Verification items for the finished model (mm, model axes). A direction names the side the tool comes from. Round coordinates to 2 decimals unless told otherwise and drop trailing zeros. Order: outer loops, then holes, each group sorted by start corner. A loop starts at its lowest first (then second) coordinate and runs counter-clockwise, first axis right, second up. Notation, with made-up numbers: (73.25, 11.25) -> (114.25, 11.25) arc R7 ccw to (114.25, 23.25) -> close; hole circle Ø4 at (-23, 53). An arc over 180 degrees is marked (long way). Put each result on its own line as item: value.
```python
from build123d import *

# Parameters (mm, degrees)
SKETCH1_R           = 2.286
BOSS_EXTRUDE1_DEPTH = 6.35
CHAMFER1_SIZE       = 15.24
CHAMFER1_SIZE2      = 24.085722971
FILLET1_R           = 3.81


with BuildPart() as part:
    # Sketch1 → Boss-Extrude1 (new body)
    with BuildSketch(Plane.XY):
        Polygon((-6.35, 31.75), (-6.35, 10.18883388), (-34.206786825, -8.403439207), (-27.156560793, -18.966786825), (-6.35, -5.08), (6.35, -5.08), (6.35, 31.75), align=None)
        Circle(SKETCH1_R, mode=Mode.SUBTRACT)
        with Locations((0, 25.4)):
            Circle(SKETCH1_R, mode=Mode.SUBTRACT)
        with Locations((-25.4, -10.16)):
            Circle(SKETCH1_R, mode=Mode.SUBTRACT)
        with Locations((0, 12.7)):
            Circle(SKETCH1_R, mode=Mode.SUBTRACT)
    extrude(amount=BOSS_EXTRUDE1_DEPTH)

    # Chamfer1
    chamfer1_edges = [part.edges().sort_by_distance(p)[0] for p in [
        (-6.35, 10.18883388, 3.175),
    ]]
    chamfer1_side = [part.faces().sort_by_distance(p)[0] for p in [
        (-6.35, 20.96941694, 3.175),
    ]]
    chamfer(chamfer1_edges, length=CHAMFER1_SIZE, length2=CHAMFER1_SIZE2, reference=chamfer1_side[0])

    # Fillet1
    fillet1_edges = [part.edges().sort_by_distance(p)[0] for p in [
        (6.35, 31.75, 3.175),
        (6.35, -5.08, 3.175),
        (-6.35, -5.08, 3.175),
        (-27.156560793, -18.966786825, 3.175),
        (-34.206786825, -8.403439207, 3.175),
        (-6.35, 31.75, 3.175),
        (-26.383532628, -3.182015811, 3.175),
        (-6.35, 25.42883388, 3.175),
    ]]
    fillet(fillet1_edges, radius=FILLET1_R)


solid = part.part
```
Item 1: Sectioned sample at C-C, the plane y = -10.16. Record the boundary of the cut face in (x, z), then the cut area to 3 significant figures.
Geometry check:
outline: (-32.67, 0) -> (-27.69, 0) -> (-27.69, 6.35) -> (-32.67, 6.35) -> close; (-23.11, 0) -> (-13.96, 0) -> (-13.96, 6.35) -> (-23.11, 6.35) -> close
area: 89.8 mm2
Item 2: Sectioned sample at A-A, the plane x = 0. Record the boundary of the cut face in (y, z), then the cut area to 3 significant figures.
Geometry check:
outline: (-5.08, 0) -> (-2.29, 0) -> (-2.29, 6.35) -> (-5.08, 6.35) -> close; (2.29, 0) -> (10.41, 0) -> (10.41, 6.35) -> (2.29, 6.35) -> close; (14.99, 0) -> (23.11, 0) -> (23.11, 6.35) -> (14.99, 6.35) -> close; (27.69, 0) -> (31.75, 0) -> (31.75, 6.35) -> (27.69, 6.35) -> close
area: 147 mm2
Item 3: Sectioned sample at B-B, the plane z = 2.25. Record the boundary of the cut face in (x, y), then the cut area to 3 significant figures.
Geometry check:
outline: (-32.09, -11.57) -> (-29.27, -15.8) arc R3.81 ccw to (-23.99, -16.85) -> (-7.31, -5.72) arc R3.81 cw to (-5.2, -5.08) -> (2.54, -5.08) arc R3.81 ccw to (6.35, -1.27) -> (6.35, 27.94) arc R3.81 ccw to (2.54, 31.75) -> (-2.54, 31.75) arc R3.81 ccw to (-6.35, 27.94) -> (-6.35, 26.63) arc R3.81 cw to (-7.04, 24.44) -> (-25.97, -2.6) arc R3.81 cw to (-26.98, -3.58) -> (-31.04, -6.29) arc R3.81 ccw to start; hole circle Ø4.57 at (-25.4, -10.16); hole circle Ø4.57 at (0, 0); hole circle Ø4.57 at (0, 12.7); hole circle Ø4.57 at (0, 25.4)
area: 911 mm2
Item 4: Material ranges on line 1 along Y through (x, z) = (0, 4.75); line 2 along Y through (x, z) = (1, 4); line 3 along X through (y, z) = (27, 0.5), recorded low to high.
Geometry check:
line 1: -5.08 to -2.29, 2.29 to 10.41, 14.99 to 23.11, 27.69 to 31.75
line 2: -5.08 to -2.06, 2.06 to 10.64, 14.76 to 23.34, 27.46 to 31.75
line 3: -6.35 to -1.63, 1.63 to 6.35
Item 5: Release check for a two-part mould opening along Y. For faces 4 (the face through (-6.52, 25.5, 3.22)), 5 (the face through (6.35, 13, 3)), 6 (the face through (-24.35, -12.19, 3.13)) record: pulls with the +Y half, pulls with the -Y half, needs draft (parallel to the pull), parting line crosses it, or undercut.
Geometry check:
face 4: pulls with the +Y half
face 5: needs draft
face 6: undercut
Item 6: Tool access check on faces 1 (the face through (-6.35, 27, 3)), 2 (the face through (-30.7, -13.66, 3.13)), 3 (the face through (-1, -5.08, 3)). Record the directions out of +Z, -Z, +X, -X, +Y, -Y that give a thin tool (end or side, any length) a straight path to the whole face; none if there is none.
Geometry check:
face 1: +Z, -Z, -X, +Y
face 2: +Z, -Z, -X, -Y
face 3: +Z, -Z, +X, -Y
Item 7: Sectioned sample at D-D, the plane y = 14. Record the boundary of the cut face in (x, z).
Geometry check:
outline: (-14.35, 0) -> (-1.88, 0) -> (-1.88, 6.35) -> (-14.35, 6.35) -> close; (1.88, 0) -> (6.35, 0) -> (6.35, 6.35) -> (1.88, 6.35) -> close
Item 8: Depth check by flat-ended pin: pin 1 Ø1.5 at (x, z) = (-27, 2.5) entering from +Y; pin 2 Ø1.5 at (y, z) = (17, 2.5) entering from -X; pin 3 Ø3 at (y, z) = (-2, 5) entering from -X. Enter the tip coordinate at first touch or a pass-through.
Geometry check:
pin 1: y = -2.95
pin 2: x = -12.78
pin 3: x = -26.86
